Print and shaded views of the part. All mm, measured from the part's lowest x, y and z. A direction names the side the tool comes from. Round coordinates to 2 decimals unless told otherwise and drop trailing zeros. Write each loop counter-clockwise with the first axis right and the second up, starting at its lowest first coordinate (ties: lowest second). Pieces come first, ordered by that corner, then holes.
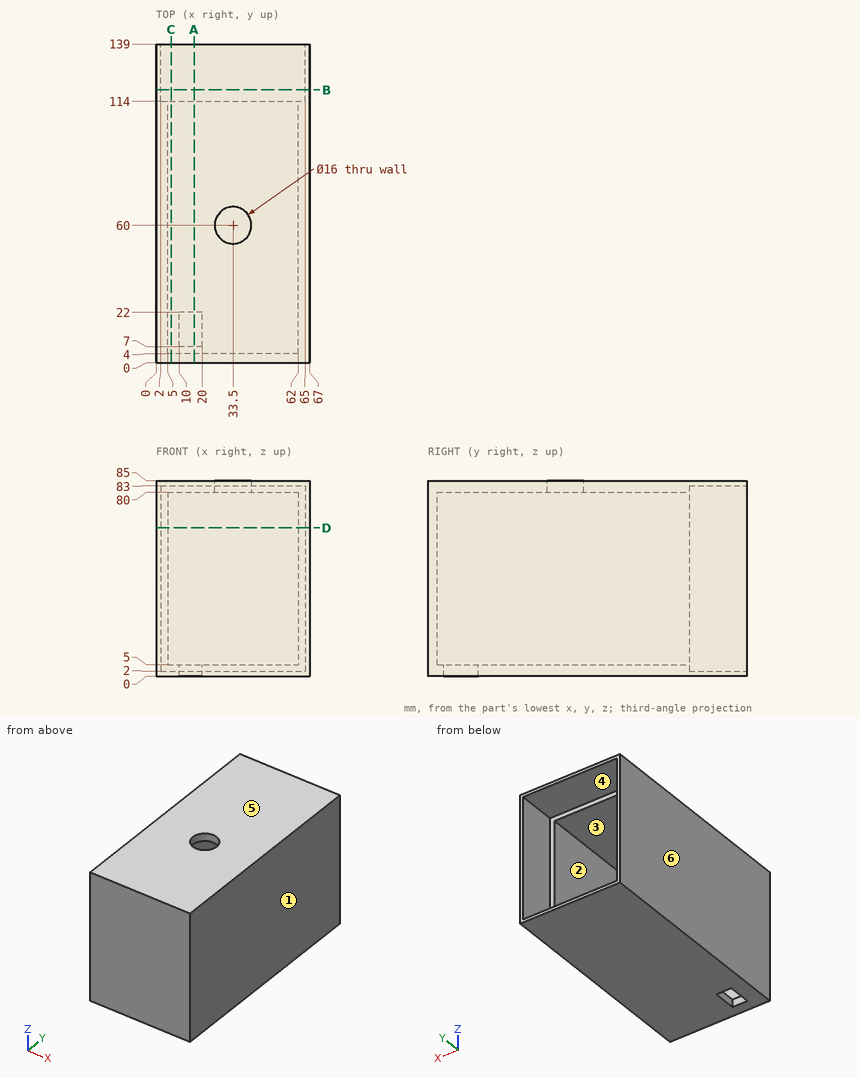
1) Slice it at C-C (x = 6.5). Write the cut outline in (y, z), plus the area to 3 significant figures.
Results:
outline: (0, 0) - (139, 0) - (139, 2) - (114, 2) - (114, 5) - (4, 5) - (4, 80) - (114, 80) - (114, 83) - (139, 83) - (139, 85) - (0, 85) - close
area: 1,540 mm2
2) Slice it at B-B (y = 119). Write the cut outline in (x, z).
Results:
outline: (0, 0) - (67, 0) - (67, 85) - (0, 85) - close; hole (2, 2) - (65, 2) - (65, 83) - (2, 83) - close
3) Pin check, flat tip, straight feed: pin 1 Ø19 at (x, z) = (37, 29) entering from +Y. Stop position of the tip, or through.
Results:
pin 1: stops at y = 4
4) Wall check: L1, parallel to Z at x = 19, y = 67.5; L2, parallel to Y at x = 33.5, z = 81.6; L3, parallel to X at y = 18, z = 73. Give the ranges that are in metal, low to high.
Results:
L1: z = 0 to 5, 80 to 85
L2: y = 0 to 52, 68 to 114
L3: x = 0 to 5, 62 to 67
5) Slice it at D-D (z = 64.5). Write the cut outline in (x, y).
Results:
outline: (0, 0) - (67, 0) - (67, 139) - (65, 139) - (65, 114) - (62, 114) - (62, 4) - (5, 4) - (5, 114) - (2, 114) - (2, 139) - (0, 139) - close
6) Which spindle directions (+Z, -Z, +X, -X, +Y, -Y) get a long thin tool onto all of the face, cutting with end or side? Do the marked faces 1 and 2. Say none if no direction does.
Results:
face 1: +Z, -Z, +X, +Y, -Y
face 2: +Y
7) Slice it at A-A (x = 16.5). Write the cut outline in (y, z).
Results:
outline: (0, 0) - (7, 0) - (7, 5) - (4, 5) - (4, 80) - (114, 80) - (114, 83) - (139, 83) - (139, 85) - (0, 85) - close; (22, 0) - (139, 0) - (139, 2) - (114, 2) - (114, 5) - (22, 5) - close
8) Mould opens along X. For the marked faces 3, 4, 5 and 6 say: released by +X, released by -X, zero draft, split by the parting line, or undercut.
Results:
face 3: undercut
face 4: undercut
face 5: zero draft
face 6: released by -X
